from build123d import *

# Parameters (mm, degrees)
F0_R     = 152.4
F0_R_2   = 127
F1_DEPTH = 3
F2_W     = 5.139328
F2_H     = 12.614713
F3_DEPTH = 25.4


with BuildPart() as f1:
    # F0 (on Top) → F1 (new body)
    with BuildSketch(Plane.XY):
        Circle(F0_R)
        Circle(F0_R_2, mode=Mode.SUBTRACT)
    extrude(amount=F1_DEPTH)

    # F2 (on face) → F3 (cut)
    with BuildSketch(Plane.XY.offset(3)):
        Polygon((-106.028961, 75.65495), (-116.953622, 81.962306), (-119.523286, 77.511517), (-108.598625, 71.204161), align=None)
        Polygon((118.533589, 53.996299), (129.45825, 60.303655), (126.888586, 64.754444), (115.963925, 58.447088), align=None)
        with Locations((-9.934964, -135.958604)):
            Rectangle(F2_W, F2_H)
    extrude(amount=-F3_DEPTH, mode=Mode.SUBTRACT)


solid = f1.part
Can you work these out from the model? Positions are in its coordinate system, mm. Give positions to 0.01 mm unless a question says otherwise; leave off trailing zeros. Write each loop counter-clockwise with the first axis right and the second up, starting at its lowest first coordinate (ties: lowest second). Pieces come first, ordered by that corner, then holes. Notation, with made-up numbers: M 28.5,-3.5 L 57.5,-3.5 A25 cw 57.5,17.5 Z; hole C -35,-36 d2. An arc over 180 degrees is marked long. Answer in a Markdown table with one row per item. Add a question column.
Item 1: Imagine slicing it at C-C, the plane z = 1.65. Write out the boundary of the cut face in (x, y), plus the area to 3 significant figures.
Item 2: Please list where these lines run through material, in increasing order: L1, parallel to Y at x = 0, z = 1.5; L2, parallel to X at y = 60, z = 0.8; L3, parallel to X at y = -75, z = 0.55.
Item 3: Imagine slicing it at A-A, the plane y = 0. Write out the boundary of the cut face in (x, z), plus the area to 3 significant figures.
Item 4: We'd pull the mould along X, two halves only. Please class faces 1 (the cylindrical face through (-120.94, -92.73, 1.48)), 2 (the cylindrical face through (-27.53, -123.98, 1.48)), 3 (the flat face through (-57, 114, 3)): released by +X, released by -X, zero draft, split by the parting line, or undercut.
Item 5: For pin 1 Ø0.9 at (x, z) = (-10, 2) entering from +Y; pin 2 Ø1 at (y, z) = (-116.5, 0.5) entering from +X; pin 3 Ø1.5 at (x, z) = (-115, 1) entering from -Y, each with a flat end and sliding along its axis, tell me the tip position at first contact or that it passes through.
Evaluation:
| question | item | result |
|---|---|---|
| 1 | outline | C 0,0 d304.8; hole C 0,0 d254; hole M -119.52,77.51 L -108.6,71.2 L -106.03,75.65 L -116.95,81.96 Z; hole M -12.5,-142.27 L -7.37,-142.27 L -7.37,-129.65 L -12.5,-129.65 Z; hole M 115.96,58.45 L 118.53,54 L 129.46,60.3 L 126.89,64.75 Z |
| 1 | area | 22,100 mm² |
| 2 | L1 | y = -152.4 to -127, 127 to 152.4 |
| 2 | L2 | x = -140.09 to -111.93, 111.93 to 118.65, 128.93 to 140.09 |
| 2 | L3 | x = -132.67 to -102.49, 102.49 to 132.67 |
| 3 | outline | M -152.4,0 L -127,0 L -127,3 L -152.4,3 Z; M 127,0 L 152.4,0 L 152.4,3 L 127,3 Z |
| 3 | area | 152 mm² |
| 4 | face 1 | split by the parting line |
| 4 | face 2 | undercut |
| 4 | face 3 | zero draft |
| 5 | pin 1 | stops at y = 152.1 |
| 5 | pin 2 | stops at x = 98.84 |
| 5 | pin 3 | stops at y = -100.86 |
